```python
from build123d import *

# Parameters (mm, degrees)
F0_R        = 1.8
F0_W        = 13.3
F0_H        = 10
F0_R_2      = 2.15
F1_DEPTH    = 7.9
F2_R        = 2.575
F2_R_2      = 5.5
F2_W        = 13.3
F2_H        = 10
F2_R_3      = 2.15
F3_DEPTH    = 4.7
F4_T1_DEPTH = 4.7
F5_T1_DEPTH = 37.6
F6_SIZE     = 0.6
F7_SIZE2    = 0.25
F7_SIZE     = 3.7
F7_2_SIZE2  = 0.25
F7_2_SIZE   = 3.7
F7_3_SIZE2  = 0.25
F7_3_SIZE   = 3.7
F8_DEPTH    = 5
F9_R        = 7.1
F9_R_2      = 5.5
F10_DEPTH   = 4.2
F9_R_3      = 4.5
F11_DEPTH   = 4.2
F12_SIZE    = 0.3
F12_2_SIZE  = 0.3
F13_R       = 5.5
F13_R_2     = 2.1
F14_DEPTH   = 0.3
F16_DEPTH   = 3


# Not quite as in the source:
# - a fillet or chamfer that OpenCascade refuses, or shapes differently, is made with other operations: its cross-section is extruded or revolved along the edge and cut away or added


with BuildPart() as f1:
    # F0 (on Top) → F1 (new body)
    with BuildSketch(Plane.XY):
        Polygon((-10.5, 10.5), (6, 10.5), (6, 25), (-25, 25), (-25, 19), (-25, 9), (-25, -9), (-25, -19), (-25, -25), (-8, -25), (-8, -10.5), (-10.5, -10.5), align=None)
        with Locations((-15.475, -8.9344954157)):
            Circle(F0_R, mode=Mode.SUBTRACT)
        with Locations((0, 17.8689908314)):
            Circle(F0_R, mode=Mode.SUBTRACT)
        with Locations((-31.65, 14)):
            Rectangle(F0_W, F0_H)
        with Locations((-33, 14)):
            Circle(F0_R_2, mode=Mode.SUBTRACT)
        with Locations((-31.65, -14)):
            Rectangle(F0_W, F0_H)
        with Locations((-33, -14)):
            Circle(F0_R_2, mode=Mode.SUBTRACT)
    extrude(amount=F1_DEPTH)



with BuildPart() as f1b:
    # F0 (on Top) → F1, piece 2 (new body)
    with BuildSketch(Plane.XY):
        Polygon((8, 10.5), (10.5, 10.5), (10.5, -10.5), (-6, -10.5), (-6, -25), (25, -25), (25, -19), (25, -9), (25, 9), (25, 19), (25, 25), (8, 25), align=None)
        with Locations((15.475, -8.9344954157)):
            Circle(F0_R, mode=Mode.SUBTRACT)
        with Locations((31.65, -14)):
            Rectangle(F0_W, F0_H)
        with Locations((33, -14)):
            Circle(F0_R_2, mode=Mode.SUBTRACT)
        with Locations((31.65, 14)):
            Rectangle(F0_W, F0_H)
        with Locations((33, 14)):
            Circle(F0_R_2, mode=Mode.SUBTRACT)
    extrude(amount=F1_DEPTH)


with BuildPart() as f1_1:
    add(f1.part)

    add(f1b.part)  # F3 merges F1b
    # F2 (on face) → F3 (join)
    with BuildSketch(Plane.XY.offset(7.9)):
        Polygon((6, 10.5), (6, 25), (-25, 25), (-25, 19), (-25, 9), (-25, -9), (-25, -19), (-25, -25), (-8, -25), (-8, -10.5), (-10.5, -10.5), (-10.5, 10.5), align=None)
        with Locations((-15.475, -8.9344954157)):
            Circle(F2_R, mode=Mode.SUBTRACT)
        with Locations((0, 17.8689908314)):
            Circle(F2_R, mode=Mode.SUBTRACT)
        Polygon((25, 19), (25, 25), (8, 25), (8, 10.5), (8, 5), (6, 5), (6, 10.5), (-10.5, 10.5), (-10.5, -10.5), (-8, -10.5), (-8, -5), (-6, -5), (-6, -10.5), (-6, -25), (25, -25), (25, -19), (25, -9), (25, 9), align=None)
        with Locations((15.475, -8.9344954157)):
            Circle(F2_R, mode=Mode.SUBTRACT)
        Circle(F2_R_2, mode=Mode.SUBTRACT)
        with Locations((-31.65, -14)):
            Rectangle(F2_W, F2_H)
        with Locations((-33, -14)):
            Circle(F2_R_3, mode=Mode.SUBTRACT)
        with Locations((-31.65, 14)):
            Rectangle(F2_W, F2_H)
        with Locations((-33, 14)):
            Circle(F2_R_3, mode=Mode.SUBTRACT)
        with Locations((31.65, 14)):
            Rectangle(F2_W, F2_H)
        with Locations((33, 14)):
            Circle(F2_R_3, mode=Mode.SUBTRACT)
        with Locations((31.65, -14)):
            Rectangle(F2_W, F2_H)
        with Locations((33, -14)):
            Circle(F2_R_3, mode=Mode.SUBTRACT)
    extrude(amount=F3_DEPTH)

    # F4: fillet of radius 1 on 4 edges, made by hand

    # F4_s2 → F4_t1 (join)
    with BuildSketch(Plane.XY.offset(7.9)):
        with BuildLine():
            ThreePointArc((-7, -5), (-6.2928932188, -5.2928932188), (-6, -6))
            Line((-6, -6), (-6, -5))
            Line((-6, -5), (-7, -5))
        make_face()
        with BuildLine():
            ThreePointArc((-8, -6), (-7.7071067812, -5.2928932188), (-7, -5))
            Line((-7, -5), (-8, -5))
            Line((-8, -5), (-8, -6))
        make_face()
        with BuildLine():
            ThreePointArc((6, 6), (6.2928932188, 5.2928932188), (7, 5))
            Line((7, 5), (6, 5))
            Line((6, 5), (6, 6))
        make_face()
        with BuildLine():
            ThreePointArc((7, 5), (7.7071067812, 5.2928932188), (8, 6))
            Line((8, 6), (8, 5))
            Line((8, 5), (7, 5))
        make_face()
    extrude(amount=F4_T1_DEPTH)

    # F5: fillet of radius 5 on 16 edges, made by hand

    # F5_s2 → F5_t1 (cut)
    with BuildSketch(Plane.XY.offset(-12.5)):
        with BuildLine():
            ThreePointArc((-38.3, 14), (-36.8355339059, 10.4644660941), (-33.3, 9))
            Line((-33.3, 9), (-38.3, 9))
            Line((-38.3, 9), (-38.3, 14))
        make_face()
        with BuildLine():
            ThreePointArc((-33.3, 19), (-36.8355339059, 17.5355339059), (-38.3, 14))
            Line((-38.3, 14), (-38.3, 19))
            Line((-38.3, 19), (-33.3, 19))
        make_face()
        with BuildLine():
            ThreePointArc((-38.3, -14), (-36.8355339059, -17.5355339059), (-33.3, -19))
            Line((-33.3, -19), (-38.3, -19))
            Line((-38.3, -19), (-38.3, -14))
        make_face()
        with BuildLine():
            ThreePointArc((-33.3, -9), (-36.8355339059, -10.4644660941), (-38.3, -14))
            Line((-38.3, -14), (-38.3, -9))
            Line((-38.3, -9), (-33.3, -9))
        make_face()
        with BuildLine():
            ThreePointArc((33.3, -19), (36.8355339059, -17.5355339059), (38.3, -14))
            Line((38.3, -14), (38.3, -19))
            Line((38.3, -19), (33.3, -19))
        make_face()
        with BuildLine():
            ThreePointArc((38.3, -14), (36.8355339059, -10.4644660941), (33.3, -9))
            Line((33.3, -9), (38.3, -9))
            Line((38.3, -9), (38.3, -14))
        make_face()
        with BuildLine():
            ThreePointArc((33.3, 9), (36.8355339059, 10.4644660941), (38.3, 14))
            Line((38.3, 14), (38.3, 9))
            Line((38.3, 9), (33.3, 9))
        make_face()
        with BuildLine():
            ThreePointArc((38.3, 14), (36.8355339059, 17.5355339059), (33.3, 19))
            Line((33.3, 19), (38.3, 19))
            Line((38.3, 19), (38.3, 14))
        make_face()
        with BuildLine():
            ThreePointArc((-25, -20), (-23.5355339059, -23.5355339059), (-20, -25))
            Line((-20, -25), (-25, -25))
            Line((-25, -25), (-25, -20))
        make_face()
        with BuildLine():
            ThreePointArc((20, -25), (23.5355339059, -23.5355339059), (25, -20))
            Line((25, -20), (25, -25))
            Line((25, -25), (20, -25))
        make_face()
        with BuildLine():
            ThreePointArc((20, 25), (23.5355339059, 23.5355339059), (25, 20))
            Line((25, 20), (25, 25))
            Line((25, 25), (20, 25))
        make_face()
        with BuildLine():
            ThreePointArc((-20, 25), (-23.5355339059, 23.5355339059), (-25, 20))
            Line((-25, 20), (-25, 25))
            Line((-25, 25), (-20, 25))
        make_face()
        with BuildLine():
            ThreePointArc((6, 20), (4.5355339059, 23.5355339059), (1, 25))
            Line((1, 25), (6, 25))
            Line((6, 25), (6, 20))
        make_face()
        with BuildLine():
            ThreePointArc((8, 20), (9.4644660941, 23.5355339059), (13, 25))
            Line((13, 25), (8, 25))
            Line((8, 25), (8, 20))
        make_face()
        with BuildLine():
            ThreePointArc((-8, -20), (-9.4644660941, -23.5355339059), (-13, -25))
            Line((-13, -25), (-8, -25))
            Line((-8, -25), (-8, -20))
        make_face()
        with BuildLine():
            ThreePointArc((-6, -20), (-4.5355339059, -23.5355339059), (-1, -25))
            Line((-1, -25), (-6, -25))
            Line((-6, -25), (-6, -20))
        make_face()
    extrude(amount=F5_T1_DEPTH, mode=Mode.SUBTRACT)

    # F6
    f6_edges = [f1_1.edges().sort_by_distance(p)[0] for p in [
        (-10.5, 0, 0),
        (-9.25, -10.5, 0),
        (2.25, -10.5, 0),
        (10.5, 0, 0),
        (9.25, 10.5, 0),
        (-2.25, 10.5, 0),
        (-6, -8.25, 7.9),
        (8, 8.25, 7.9),
        (-8, -10.5, 3.95),
        (-6, -10.5, 3.95),
        (6, 10.5, 3.95),
        (8, 10.5, 3.95),
        (7.707107, 5.292893, 7.9),
        (6.292893, 5.292893, 7.9),
        (6, 8.25, 7.9),
        (-8, -8.25, 7.9),
        (-7.707107, -5.292893, 7.9),
        (-6.292893, -5.292893, 7.9),
    ]]
    chamfer(f6_edges, length=F6_SIZE)

    # F7
    f7_edges = [f1_1.edges().sort_by_distance(p)[0] for p in [
        (-2.575, 17.868991, 12.6),
    ]]
    f7_side = f1_1.faces().sort_by_distance((-2.575, 17.868991, 10.25))[0]
    chamfer(f7_edges, length=F7_SIZE, length2=F7_SIZE2, reference=f7_side)

    # F7#2
    f7_2_edges = [f1_1.edges().sort_by_distance(p)[0] for p in [
        (12.9, -8.934495, 12.6),
    ]]
    f7_2_side = f1_1.faces().sort_by_distance((12.9, -8.934495, 10.25))[0]
    chamfer(f7_2_edges, length=F7_2_SIZE, length2=F7_2_SIZE2, reference=f7_2_side)

    # F7#3
    f7_3_edges = [f1_1.edges().sort_by_distance(p)[0] for p in [
        (-18.05, -8.934495, 12.6),
    ]]
    f7_3_side = f1_1.faces().sort_by_distance((-18.05, -8.934495, 10.25))[0]
    chamfer(f7_3_edges, length=F7_3_SIZE, length2=F7_3_SIZE2, reference=f7_3_side)

    # F0 (on Top) → F8 (cut)
    with BuildSketch(Plane.XY):
        Polygon((-10.5, 10.5), (6, 10.5), (6, 25), (-25, 25), (-25, 19), (-25, 9), (-25, -9), (-25, -19), (-25, -25), (-8, -25), (-8, -10.5), (-10.5, -10.5), align=None)
        with Locations((-15.475, -8.9344954157)):
            Circle(F0_R, mode=Mode.SUBTRACT)
        with Locations((0, 17.8689908314)):
            Circle(F0_R, mode=Mode.SUBTRACT)
        Polygon((8, 10.5), (10.5, 10.5), (10.5, -10.5), (-6, -10.5), (-6, -25), (25, -25), (25, -19), (25, -9), (25, 9), (25, 19), (25, 25), (8, 25), align=None)
        with Locations((15.475, -8.9344954157)):
            Circle(F0_R, mode=Mode.SUBTRACT)
        with Locations((-31.65, -14)):
            Rectangle(F0_W, F0_H)
        with Locations((-33, -14)):
            Circle(F0_R_2, mode=Mode.SUBTRACT)
        with Locations((-31.65, 14)):
            Rectangle(F0_W, F0_H)
        with Locations((-33, 14)):
            Circle(F0_R_2, mode=Mode.SUBTRACT)
        with Locations((31.65, 14)):
            Rectangle(F0_W, F0_H)
        with Locations((33, 14)):
            Circle(F0_R_2, mode=Mode.SUBTRACT)
        with Locations((31.65, -14)):
            Rectangle(F0_W, F0_H)
        with Locations((33, -14)):
            Circle(F0_R_2, mode=Mode.SUBTRACT)
    extrude(amount=F8_DEPTH, mode=Mode.SUBTRACT)

    # F9 (on face) → F10 (cut)
    with BuildSketch(Plane.XY.offset(12.6)):
        Circle(F9_R)
        Circle(F9_R_2, mode=Mode.SUBTRACT)
    extrude(amount=-F10_DEPTH, mode=Mode.SUBTRACT)

    # F12
    f12_edges = [f1_1.edges().sort_by_distance(p)[0] for p in [
        (-5.5, 0, 7.9),
        (-7.1, 0, 12.6),
    ]]
    chamfer(f12_edges, length=F12_SIZE)



with BuildPart() as f11:
    # F9 (on face) → F11 (new body, through all)
    with BuildSketch(Plane.XY.offset(12.6)):
        Circle(F9_R_3)
    extrude(amount=-F11_DEPTH)

    # F12#2
    f12_2_edges = [f11.edges().sort_by_distance(p)[0] for p in [
        (-4.5, 0, 12.6),
    ]]
    chamfer(f12_2_edges, length=F12_2_SIZE)


with BuildPart() as f1_2:
    add(f1_1.part)

    add(f11.part)  # F14 merges F11
    # F13 (on face) → F14 (join)
    with BuildSketch(Plane.XY.offset(8.4)):
        Circle(F13_R)
        Circle(F13_R_2, mode=Mode.SUBTRACT)
    extrude(amount=-F14_DEPTH)

    # F15 (on face) → F16 (join)
    with BuildSketch(Plane.XY.offset(12.6)):
        with BuildLine():
            Line((-6, -20), (-6, -6))
            ThreePointArc((-6, -6), (-6.2928932188, -5.2928932188), (-7, -5))
            ThreePointArc((-7, -5), (-7.7071067812, -5.2928932188), (-8, -6))
            Line((-8, -6), (-8, -20))
            Line((-8, -20), (-6, -20))
        make_face()
        with BuildLine():
            Line((8, 6), (8, 20))
            Line((8, 20), (6, 20))
            Line((6, 20), (6, 11.1))
            Line((6, 11.1), (6, 6))
            ThreePointArc((6, 6), (6.2928932188, 5.2928932188), (7, 5))
            ThreePointArc((7, 5), (7.7071067812, 5.2928932188), (8, 6))
        make_face()
    extrude(amount=-F16_DEPTH)


solid = f1_2.part
```
The listing builds one solid part. Answer for the finished solid, in the listing's coordinates (mm). A direction names the side the tool comes from. Round coordinates to 2 decimals unless told otherwise and drop trailing zeros. Loops run counter-clockwise (first coordinate to the right, second up) from the corner with the lowest first, then second, coordinate; pieces in that order, holes last. Notation, with made-up numbers: (46.25, -26) -> (71.25, -26) arc R26 ccw to (71.25, -5) -> close; hole circle Ø7 at (23.25, 30.25). An arc over 180 degrees is marked (long way). Use one line per item in the form item = value.
1. For a pull along Y with two mould halves and no side action, classify faces 5 (the conical face through (-18.174, -8.816, 10.776)), 6 (the flat face through (29, 19, 9)), 7 (the flat face through (-16, 6, 5)) as released by +Y, released by -Y, zero draft, split by the parting line, or undercut.
Answer key:
face_5 = undercut
face_6 = released by +Y
face_7 = zero draft
2. Find the intervals of material crossed by probe 1 along Y at (x, z) = (33, 8.25); probe 2 along Y at (x, z) = (-0.5, 7.25); probe 3 along X at (y, z) = (-9.5, 10.5), in increasing order. Write a range as [from, to].
Answer key:
probe_1 = [-19, -16.15], [-11.85, -9], [9, 11.85], [16.15, 19]
probe_2 = [-25, -10.5], [10.5, 16.14], [19.6, 25]
probe_3 = [-35.48, -18.1], [-12.85, 12.85], [18.1, 35.48]
3. The part is cut by section A-A on x = -29.5. Determine the outline of the cut face in (y, z).
Answer key:
outline = (-19, 5) -> (-9, 5) -> (-9, 12.6) -> (-19, 12.6) -> close; (9, 5) -> (19, 5) -> (19, 12.6) -> (9, 12.6) -> close
4. The part is cut by section B-B on z = 11.25. Give the number of separate pieces and of enclosed holes in the cut face, and give its area (3 significant figures).
Answer key:
separate_pieces = 2
enclosed_holes = 8
area = 2,700 mm²
5. Flat-ended cylindrical pins translate along their axes: pin 1 Ø0.6 at (x, z) = (-6.5, 11) entering from -Y; pin 2 Ø1 at (x, z) = (-27.5, 8) entering from +Y; pin 3 Ø0.5 at (y, z) = (-19.5, 9) entering from +X; pin 4 Ø5.5 at (x, y) = (16.5, -8) entering from +Z. Find the tip coordinate at first contact, or state that the pin passes through.
Answer key:
pin_1 = -20
pin_2 = 19
pin_3 = 25
pin_4 = 12.6
6. A tool of negligible diameter and unlimited length cuts with its end or side. For faces 1 (the flat face through (-0.1, -2.4, 8.1)), 2 (the cylindrical face through (-0.92, 7.04, 10.38)), 3 (the flat face through (-29, 9, 9)), 4 (the flat face through (25, 0, 9)), from which of +Z, -Z, +X, -X, +Y, -Y can it reach the whole face along a straight path? Write none if from no direction.
Answer key:
face_1 = -Z
face_2 = +Z
face_3 = +Z, -Z, -X
face_4 = +Z, -Z, +X
